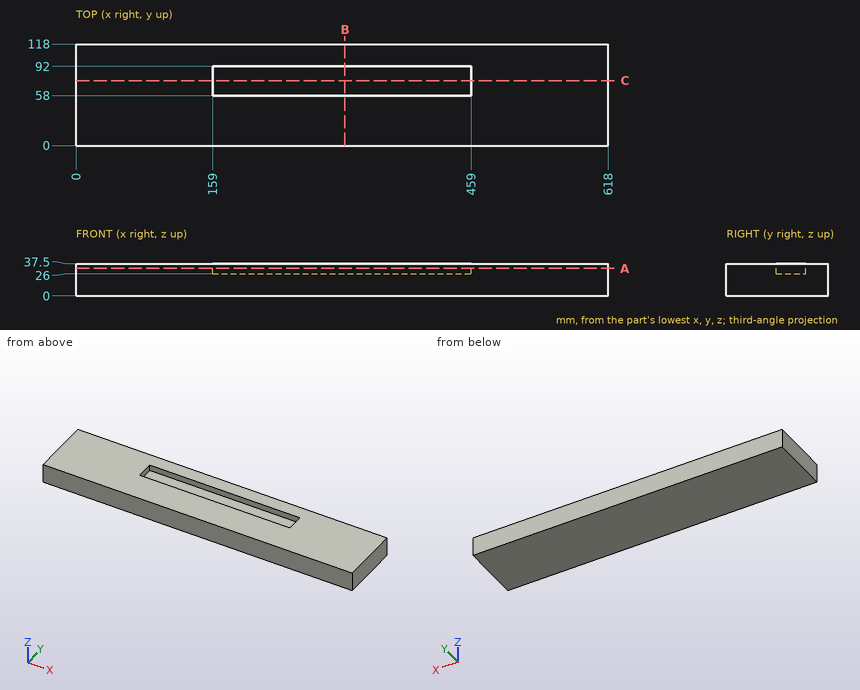
Verification items for this drawing (mm, ordinates from the low corner). Give positions to 0.01 mm unless a question says otherwise; leave off trailing zeros. Order: outer loops, then holes, each group sorted by start corner. A loop starts at its lowest first (then second) coordinate and runs counter-clockwise, first axis right, second up. Notation, with made-up numbers: M 25.25,8.5 L 76.25,8.5 A27 cw 76.25,40.5 Z; hole C -35,54.5 d8. An arc over 180 degrees is marked long. Use a Markdown table: item, result.
Item 1: Material ranges on line 1 along Y through (x, z) = (255, 36.5); line 2 along Z through (x, y) = (280, 71.5), recorded low to high.
Answers follow:
| item | result |
|---|---|
| line 1 | y = 0 to 58, 92 to 118 |
| line 2 | z = 0 to 26 |
Item 2: Depth check by flat-ended pin: P1, Ø2, axis at x = 173, y = 59.5, coming from the -Z side; P2, Ø17, axis at x = 292, y = 80.5, coming from the +Z side. Enter the tip coordinate at first touch or a pass-through.
Answers follow:
| item | result |
|---|---|
| P1 | stops at z = 0 |
| P2 | stops at z = 26 |
Item 3: Section check B-B (x = 312). Record the cut outline in (y, z), and give its area (3 significant figures).
Answers follow:
| item | result |
|---|---|
| outline | M 0,0 L 118,0 L 118,37.5 L 92,37.5 L 92,26 L 58,26 L 58,37.5 L 0,37.5 Z |
| area | 4,030 mm2 |
Item 4: Section check A-A (z = 32). Record the cut outline in (x, y).
Answers follow:
| item | result |
|---|---|
| outline | M 0,0 L 618,0 L 618,118 L 0,118 Z; hole M 159,58 L 459,58 L 459,92 L 159,92 Z |
Item 5: Section check C-C (y = 75.5). Record the cut outline in (x, z), and give its area (3 significant figures).
Answers follow:
| item | result |
|---|---|
| outline | M 0,0 L 618,0 L 618,37.5 L 459,37.5 L 459,26 L 159,26 L 159,37.5 L 0,37.5 Z |
| area | 19,700 mm2 |
